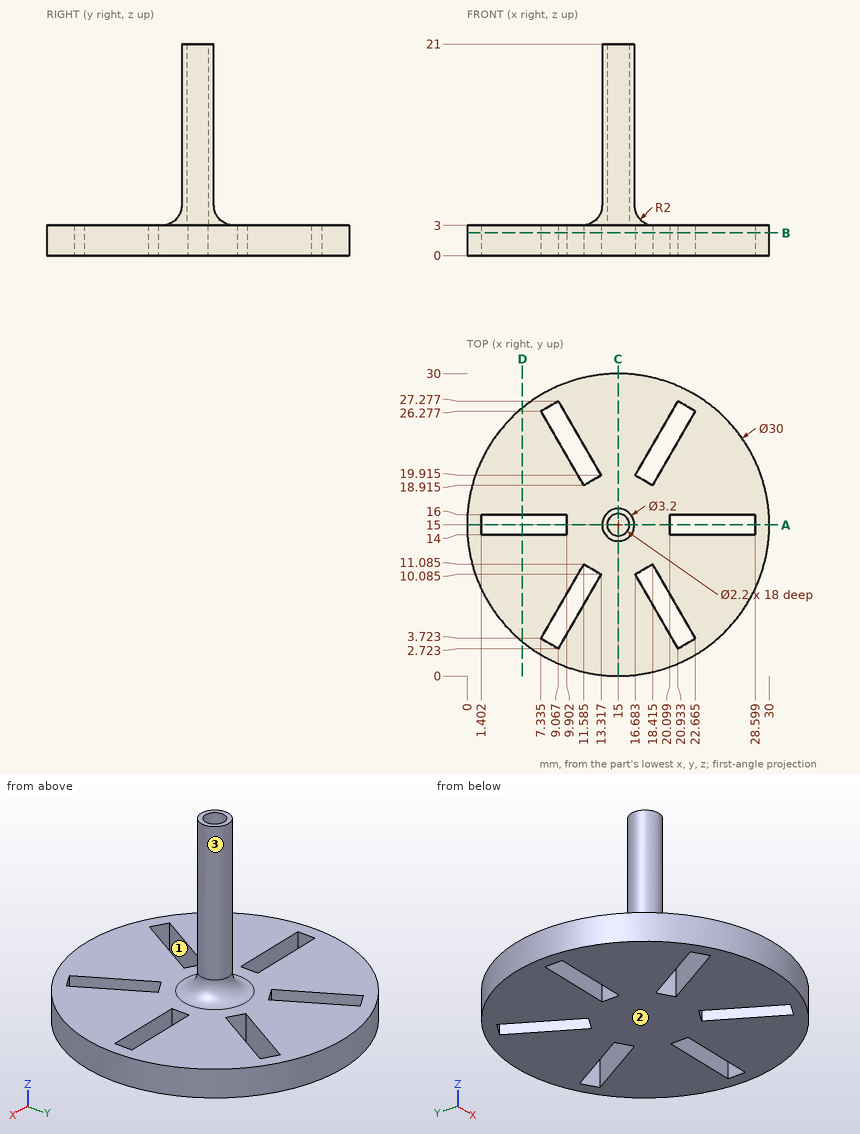
Geometry: see drawing. Coordinates: mm, zero at the bounding-box minimum. Give positions to 0.01 mm unless a question says otherwise; leave off trailing zeros. Order: outer loops, then holes, each group sorted by start corner. A loop starts at its lowest first (then second) coordinate and runs counter-clockwise, first axis right, second up.
1. Pin query (flat end, axial travel): pin 1 Ø12 at (x, y) = (19, 26) entering from +Z; pin 2 Ø0.9 at (x, z) = (7.5, 2) entering from +Y; pin 3 Ø1.5 at (x, z) = (4, 2) entering from -Y. Return the tip coordinate at first contact, or that it passes through.
Computed:
pin 1: stops at z = 3
pin 2: stops at y = 28.24
pin 3: stops at y = 4.05
2. Cut plane D-D (x = 5.5). Return loops of the section in (y, z).
Computed:
outline: (3.39, 0) - (14, 0) - (14, 3) - (3.39, 3) - close; (16, 0) - (26.61, 0) - (26.61, 3) - (16, 3) - close
3. Cut plane B-B (z = 2.25). Return loops of the section in (x, y) (1 decimal).
Computed:
outline: circle Ø30 at (15, 15); hole (1.4, 14) - (9.9, 14) - (9.9, 16) - (1.4, 16) - close; hole (7.3, 3.7) - (9.1, 2.7) - (13.3, 10.1) - (11.6, 11.1) - close; hole (7.3, 26.3) - (11.6, 18.9) - (13.3, 19.9) - (9.1, 27.3) - close; hole (16.7, 10.1) - (20.9, 2.7) - (22.7, 3.7) - (18.4, 11.1) - close; hole (16.7, 19.9) - (18.4, 18.9) - (22.7, 26.3) - (20.9, 27.3) - close; hole (20.1, 14) - (28.6, 14) - (28.6, 16) - (20.1, 16) - close
4. Line query: probe 1 along Y at (x, z) = (15, 8.5); probe 2 along Z at (x, y) = (25.5, 22). Output: solid intervals per line, ascending.
Computed:
probe 1: y = 13.4 to 13.9, 16.1 to 16.6
probe 2: z = 0 to 3
5. Cut plane A-A (y = 15). Return loops of the section in (x, z).
Computed:
outline: (0, 0) - (1.4, 0) - (1.4, 3) - (0, 3) - close; (9.9, 0) - (20.1, 0) - (20.1, 3) - (18.6, 3) arc R2 cw to (16.6, 5) - (16.6, 21) - (16.1, 21) - (16.1, 3) - (13.9, 3) - (13.9, 21) - (13.4, 21) - (13.4, 5) arc R2 cw to (11.4, 3) - (9.9, 3) - close; (28.6, 0) - (30, 0) - (30, 3) - (28.6, 3) - close
6. Draft query along Y for the marked faces 1, 2 and 3. Return one class per face: released by +Y, released by -Y, zero draft, split by the parting line, or undercut.
Computed:
face 1: undercut
face 2: zero draft
face 3: split by the parting line
7. Cut plane C-C (x = 15). Return loops of the section in (y, z), and give its area (3 significant figures).
Computed:
outline: (0, 0) - (30, 0) - (30, 3) - (18.6, 3) arc R2 cw to (16.6, 5) - (16.6, 21) - (16.1, 21) - (16.1, 3) - (13.9, 3) - (13.9, 21) - (13.4, 21) - (13.4, 5) arc R2 cw to (11.4, 3) - (0, 3) - close
area: 110 mm2
